Build history of the part. All positions in model axes, mm. A direction names the side the tool comes from. Round coordinates to 2 decimals unless told otherwise and drop trailing zeros. Loops run counter-clockwise (first coordinate to the right, second up) from the corner with the lowest first, then second, coordinate; pieces in that order, holes last.
from build123d import *

# Parameters (mm, degrees)
BOSS_EXTRUDE2_DEPTH                  = 69.85
F_10_CLEARANCE_HOLE1_D               = 5.1054
CUT_EXTRUDE1_DEPTH                   = 158.914682345
F_25_32_0_78125_DIAMETER_HOLE1_D     = 19.84375
F_25_32_0_78125_DIAMETER_HOLE1_DEPTH = 9.278336046
F_25_32_0_78125_DIAMETER_HOLE1_TIP   = 5.961663954
CONVERT_SOLID1_START                 = -69.85
CONVERT_SOLID1_DEPTH                 = 69.85
CONVERT_SOLID1_2_DEPTH               = 69.85


# Read off the part's stored shape, not the designer's step: Convert-Solid1
with BuildPart() as part:
    # Sketch8 → Boss-Extrude2 (new body)
    with BuildSketch(Plane.XY):
        Polygon((0, 2.54), (0, 0), (78.74, 0), (78.74, 119.38), (76.2, 119.38), (76.2, 2.54), align=None)
    extrude(amount=-BOSS_EXTRUDE2_DEPTH)

    # #10 Clearance Hole1 (through all)
    with Locations(Plane(origin=(0, 2.54, 0), x_dir=(1, 0, 0), z_dir=(0, 1, 0))):
        with Locations((25.4, 9.525), (25.4, 60.325)):
            Hole(F_10_CLEARANCE_HOLE1_D / 2)

    # E → Cut-Extrude1 (cut, through all)
    with BuildSketch(Plane.ZY.offset(-76.2)):
        with BuildLine():
            Line((-53.7845, 106.68), (-53.7845, 55.88))
            ThreePointArc((-53.7845, 55.88), (-57.15, 52.5145), (-60.5155, 55.88))
            Line((-60.5155, 55.88), (-60.5155, 106.68))
            ThreePointArc((-60.5155, 106.68), (-57.15, 110.0455), (-53.7845, 106.68))
        make_face()
        with BuildLine():
            Line((-9.3345, 106.68), (-9.3345, 55.88))
            ThreePointArc((-9.3345, 55.88), (-12.7, 52.5145), (-16.0655, 55.88))
            Line((-16.0655, 55.88), (-16.0655, 106.68))
            ThreePointArc((-16.0655, 106.68), (-12.7, 110.0455), (-9.3345, 106.68))
        make_face()
    extrude(amount=-CUT_EXTRUDE1_DEPTH, mode=Mode.SUBTRACT)

    # 25/32 (0.78125) Diameter Hole1
    with Locations(Plane(origin=(0, 2.54, 0), x_dir=(1, 0, 0), z_dir=(0, 1, 0))):
        with Locations((25.4, 34.925)):
            Hole(F_25_32_0_78125_DIAMETER_HOLE1_D / 2, depth=F_25_32_0_78125_DIAMETER_HOLE1_DEPTH)
            with Locations((0, 0, -(F_25_32_0_78125_DIAMETER_HOLE1_DEPTH + F_25_32_0_78125_DIAMETER_HOLE1_TIP / 2))):  # 118° drill point
                Cone(0, F_25_32_0_78125_DIAMETER_HOLE1_D / 2, F_25_32_0_78125_DIAMETER_HOLE1_TIP, mode=Mode.SUBTRACT)

    # Convert-Solid1 outline → Convert-Solid1 (cut)
    with BuildSketch(Plane.XY.offset(CONVERT_SOLID1_START)):
        with BuildLine():
            ThreePointArc((78.74, 5.08), (77.252102448, 1.487897552), (73.66, 0))
            Line((73.66, 0), (78.74, 0))
            Line((78.74, 0), (78.74, 5.08))
        make_face()
    extrude(amount=CONVERT_SOLID1_DEPTH, mode=Mode.SUBTRACT)

    # Convert-Solid1 2 outline → Convert-Solid1 2 (add)
    with BuildSketch(Plane.XY.offset(CONVERT_SOLID1_START)):
        with BuildLine():
            ThreePointArc((76.2, 5.08), (75.456051224, 3.283948776), (73.66, 2.54))
            Line((73.66, 2.54), (76.2, 2.54))
            Line((76.2, 2.54), (76.2, 5.08))
        make_face()
    extrude(amount=CONVERT_SOLID1_2_DEPTH)


solid = part.part
(1) Probe line 1 (Z direction, x = 25.4, y = 2); line 2 (Z direction, x = 25, y = 1); line 3 (Y direction, x = 39, z = -5). List the from-to ranges inside material, lowest first.
Responses:
line 1: z = -69.85 to -62.88, -57.77 to -44.85, -25 to -12.08, -6.97 to 0
line 2: z = -69.85 to -62.85, -57.8 to -44.84, -25.01 to -12.05, -7 to 0
line 3: y = 0 to 2.54
(2) Slice it at D-D on y = 50. List the corners of the cut face in (x, z), plus the area to 3 significant figures.
Responses:
outline: (76.2, -69.85) - (78.74, -69.85) - (78.74, 0) - (76.2, 0) - close
area: 177 mm2
(3) Slice it at A-A on x = 25.4. List the corners of the cut face in (y, z).
Responses:
outline: (0, -69.85) - (2.54, -69.85) - (2.54, -62.88) - (0, -62.88) - close; (0, -57.77) - (2.54, -57.77) - (2.54, -44.85) - (0, -44.85) - close; (0, -25) - (2.54, -25) - (2.54, -12.08) - (0, -12.08) - close; (0, -6.97) - (2.54, -6.97) - (2.54, 0) - (0, 0) - close
(4) Which spindle directions (+Z, -Z, +X, -X, +Y, -Y) get a long thin tool onto all of the face, cutting with end or side? Do faces 5 (the face through (78.74, 61, -34)), 6 (the face through (77, 81, -16.066)), 7 (the face through (37, 2.54, -34)). Say none if no direction does.
Responses:
face 5: +Z, -Z, +X, +Y, -Y
face 6: +X, -X
face 7: +Z, -Z, -X, +Y
(5) Slice it at B-B on z = -40. List the corners of the cut face in (x, y).
Responses:
outline: (0, 0) - (16.87, 0) - (16.87, 2.54) - (0, 2.54) - close; (33.93, 0) - (73.66, 0) arc R5.08 ccw to (78.74, 5.08) - (78.74, 119.38) - (76.2, 119.38) - (76.2, 5.08) arc R2.54 cw to (73.66, 2.54) - (33.93, 2.54) - close
(6) Slice it at C-C on z = -23. List the corners of the cut face in (x, y).
Responses:
outline: (0, 0) - (73.66, 0) arc R5.08 ccw to (78.74, 5.08) - (78.74, 119.38) - (76.2, 119.38) - (76.2, 5.08) arc R2.54 cw to (73.66, 2.54) - (0, 2.54) - close
(7) Pull direction Y, two halves, no side cores. Call faces 1 (the face through (20.822, 1.252, -26.123)), 2 (the face through (75.476, 3.304, -35.414)), 3 (the face through (77.452, 110.045, -12.774)), 4 (the face through (36, 0, -34)): +Y half, -Y half, draft (parallel to the pull), parting line (faces both ways), or undercut.
Responses:
face 1: draft
face 2: +Y half
face 3: undercut
face 4: -Y half
